Drawing for the job (mm, zero at the part's lowest x, y, z). A direction names the side the tool comes from. Give positions to 0.01 mm unless a question says otherwise; leave off trailing zeros. Write each loop counter-clockwise with the first axis right and the second up, starting at its lowest first coordinate (ties: lowest second). Pieces come first, ordered by that corner, then holes. Notation, with made-up numbers: (33, -2) - (77, -2) arc R3 ccw to (77, 2) - close; hole circle Ø10 at (13, 44). An arc over 180 degrees is marked (long way). Use CSV: the item, a comma, the result in double quotes.
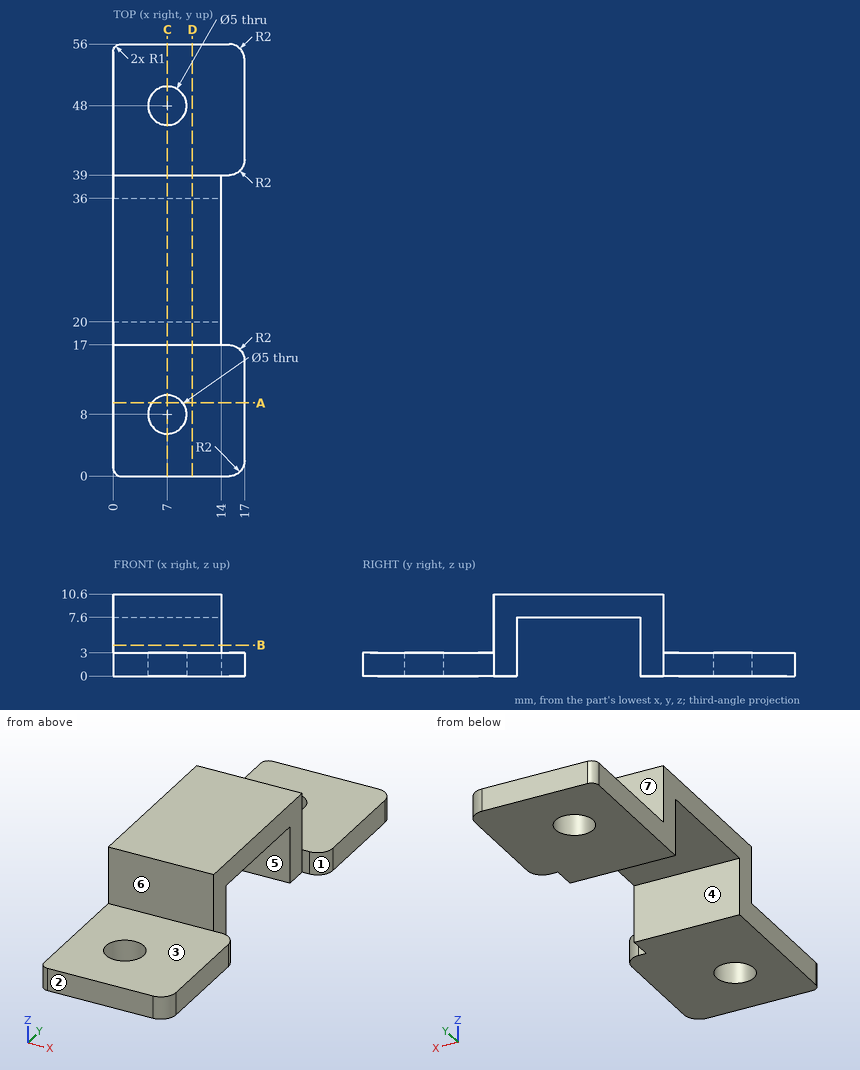
(1) Saw through at D-D, the plane x = 10.25. List the corners of the cut face in (y, z), then the cut area to 3 significant figures.
Checked values:
outline,"(0, 0) - (20, 0) - (20, 7.6) - (36, 7.6) - (36, 0) - (56, 0) - (56, 3) - (39, 3) - (39, 10.6) - (17, 10.6) - (17, 3) - (0, 3) - close"
area,"214 mm^2"
(2) Saw through at A-A, the plane y = 9.5. List the corners of the cut face in (x, z).
Checked values:
outline,"(0, 0) - (5, 0) - (5, 3) - (0, 3) - close; (9, 0) - (17, 0) - (17, 3) - (9, 3) - close"
(3) Saw through at B-B, the plane z = 4. List the corners of the cut face in (x, y).
Checked values:
outline,"(0, 17) - (14, 17) - (14, 20) - (0, 20) - close; (0, 36) - (14, 36) - (14, 39) - (0, 39) - close"
(4) Pull direction Y, two halves, no side cores. Call the marked faces 4, 5, 6 and 7: released by +Y, released by -Y, zero draft, split by the parting line, or undercut.
Checked values:
face 4,"undercut"
face 5,"undercut"
face 6,"released by -Y"
face 7,"released by +Y"
(5) Saw through at C-C, the plane x = 7. List the corners of the cut face in (y, z).
Checked values:
outline,"(0, 0) - (5.5, 0) - (5.5, 3) - (0, 3) - close; (10.5, 0) - (20, 0) - (20, 7.6) - (36, 7.6) - (36, 0) - (45.5, 0) - (45.5, 3) - (39, 3) - (39, 10.6) - (17, 10.6) - (17, 3) - (10.5, 3) - close; (50.5, 0) - (56, 0) - (56, 3) - (50.5, 3) - close"
(6) Wall check: probe 1 along Y at (x, z) = (7, 1.7); probe 2 along Y at (x, z) = (6.5, 6); probe 3 along Y at (x, z) = (1.5, 1.75). Give the ranges that are in metal, low to high. Write a range as [from, to].
Checked values:
probe 1,"y = [0, 5.5], [10.5, 20], [36, 45.5], [50.5, 56]"
probe 2,"y = [17, 20], [36, 39]"
probe 3,"y = [0, 20], [36, 56]"
(7) Flat gauge pins, fed straight in: P1, Ø6, axis at x = 7, y = 8, coming from the +Z side; P2, Ø8, axis at x = 2, y = 10, coming from the -Z side; P3, Ø4, axis at x = 10, z = 5.5, coming from the -Y side; P4, Ø4, axis at y = 39, z = 9, coming from the +X side. Where does each tip first touch, or does it go through?
Checked values:
P1,"stops at z = 3"
P2,"stops at z = 0"
P3,"stops at y = 17"
P4,"stops at x = 14"
(8) 3-axis set-ups, long thin cutter, end or side, ignore diameter. For the marked faces 1, 2 and 3: which of +Z, -Z, +X, -X, +Y, -Y reach the whole face in a straight line?
Checked values:
face 1,"+Z, -Z, +X"
face 2,"+Z, -Z, +X, -X, -Y"
face 3,"+Z, +X, -X, -Y"
